Design review of the part shown in the three views and the two pictorial views. Dimensions are in mm from the part's minimum x, y and z. A direction names the side the tool comes from. Round coordinates to 2 decimals unless told otherwise and drop trailing zeros. Write each loop counter-clockwise with the first axis right and the second up, starting at its lowest first coordinate (ties: lowest second). Pieces come first, ordered by that corner, then holes. Notation, with made-up numbers: (-17, 53.25) -> (34, 53.25) arc R28 ccw to (34, 71.25) -> close; hole circle Ø6 at (13.25, 66). An arc over 180 degrees is marked (long way). Return JSON: item names as keys, results as strings. Group by question number.
1. For line 1 along X through (y, z) = (86.5, 77.5); line 2 along Y through (x, z) = (85, 13.5); line 3 along X through (y, z) = (44.5, 104.5) (1 decimal), list the stretches that pass through material, from the lowest coordinate up. Write a range as from..to.
2. Mouldability with a two-part tool opening along X and no side actions: class the marked faces 3, 4 and 5 as pulls with the +X half, pulls with the -X half, needs draft (parallel to the pull), parting line crosses it, or undercut.
3. Take a section at A-A, the plane y = 21. Write out the cut boundary in (x, z) (1 decimal).
4. Take a section at B-B, the plane y = 85. Write out the cut boundary in (x, z), then the cut area to 3 significant figures.
5. Clearance check with flat-ended pins moving along their axes: P1, Ø3, axis at y = 47, z = 17.5, coming from the -X side (1 decimal); P2, Ø4, axis at y = 89.5, z = 98.5, coming from the +X side; P3, Ø8, axis at x = 135.5, z = 120.5, coming from the +Y side. State where each tip first meets the part, or that it passes through.
6. Tool access review of the marked faces 1 and 2: name each direction out of +Z, -Z, +X, -X, +Y, -Y from which nothing blocks a thin tool from reaching the whole face with its end or side.
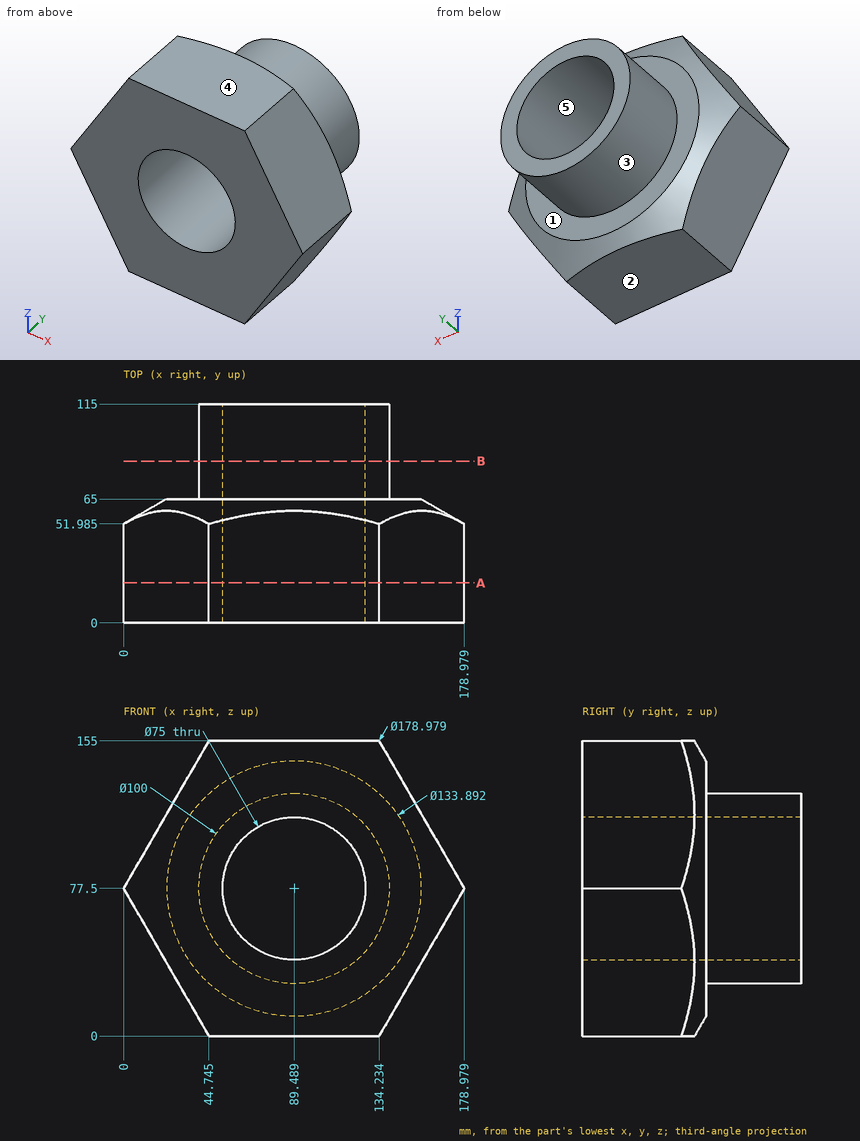
Output:
{
 "1": {"line 1": "x = 39.49..51.99, 126.99..139.49", "line 2": "y = 0..65", "line 3": "x = 15.6..63.5, 115.5..163.4"},
 "2": {"face 3": "parting line crosses it", "face 4": "needs draft", "face 5": "undercut"},
 "3": {"outline": "(0, 77.5) -> (44.7, 0) -> (134.2, 0) -> (179, 77.5) -> (134.2, 155) -> (44.7, 155) -> close; hole circle Ø75 at (89.5, 77.5)"},
 "4": {"outline": "circle Ø100 at (89.49, 77.5); hole circle Ø75 at (89.49, 77.5)", "area": "3,440 mm^2"},
 "5": {"P1": "stops at x = 33.8", "P2": "stops at x = 135.74", "P3": "stops at y = 65"},
 "6": {"face 1": "+Y", "face 2": "-Z, +X, -X, +Y, -Y"}
}
